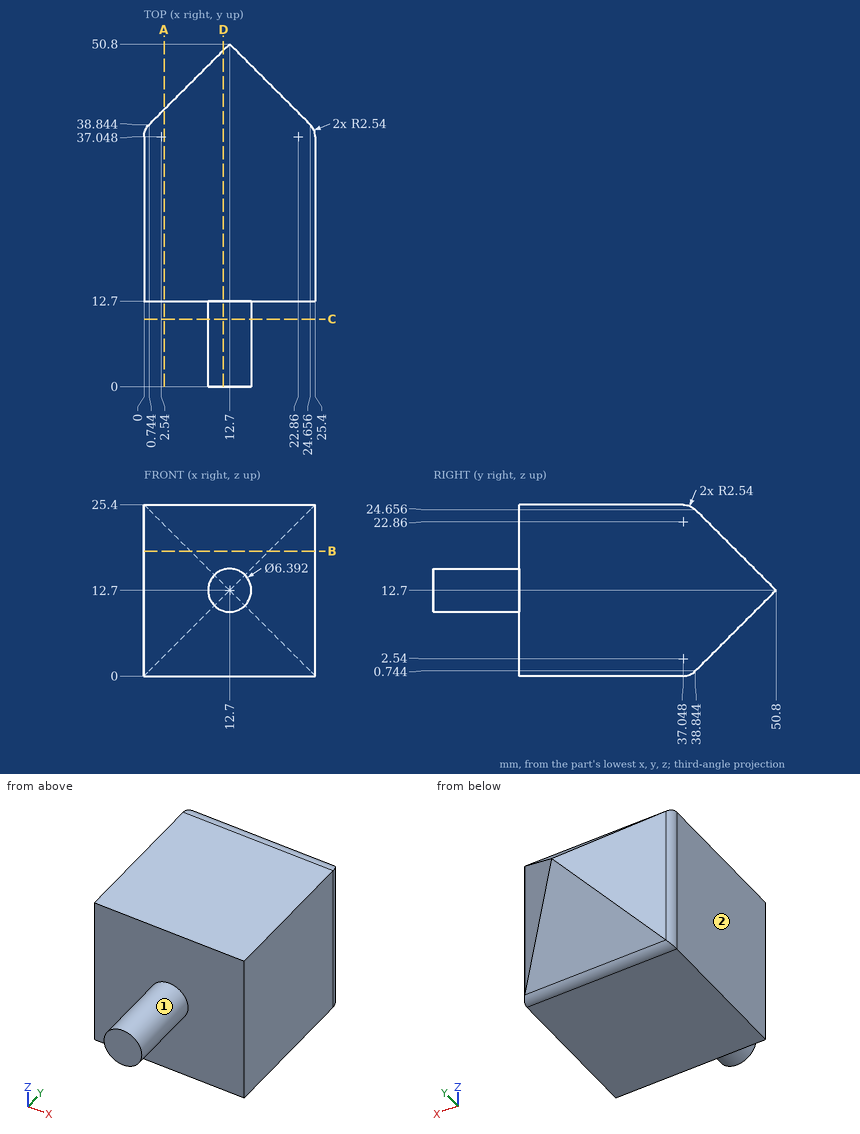
Source: three-view drawing plus pictorial views. Frame: mm from the lowest corner of the part. A direction names the side the tool comes from. Round coordinates to 2 decimals unless told otherwise and drop trailing zeros. Write each loop counter-clockwise with the first axis right and the second up, starting at its lowest first coordinate (ties: lowest second). Pieces come first, ordered by that corner, then holes. Notation, with made-up numbers: M 82.5,-34 L 130.5,-34 A18 ccw 130.5,-23 Z; hole C 9.25,5.25 d1. An arc over 180 degrees is marked long. One line per item, written item: value. Start each with the question number.
Item 1: Section query A-A (x = 3). Return the cut outline in (y, z).
Item 2: Pin query (flat end, axial travel): pin 1 (5 mm diameter, centred on x = 19.5, z = 15, fed in from -Y); pin 2 (1.5 mm diameter, centred on x = 22.5, y = 39, fed in from -Z). Return the tip coordinate at first contact, or that it passes through.
Item 3: Section query D-D (x = 11.75). Return the cut outline in (y, z).
Item 4: Section query B-B (z = 18.5). Return the cut outline in (x, y).
Item 5: Set-up query: the marked faces 1 and 2. Return all of +Z, -Z, +X, -X, +Y, -Y with unobstructed straight access to the full face (end or side cutting, diameter ignored); none if empty.
Item 6: Section query C-C (y = 10). Return the cut outline in (x, z).
Item 7: Ray query, L1, parallel to Y at x = 17, z = 23.5; L2, parallel to Z at x = 10, y = 2; L3, parallel to Y at x = 22.25, z = 1.5. Return the intervals inside material, ascending. Write a range as from..to.
Result set:
1. outline: M 12.7,0 L 37.05,0 A2.54 ccw 38.84,0.74 L 41.1,3 L 41.1,22.4 L 38.84,24.66 A2.54 ccw 37.05,25.4 L 12.7,25.4 Z
2. pin 1: stops at y = 12.7
2. pin 2: stops at z = 0.3
3. outline: M 0,9.65 L 12.7,9.65 L 12.7,0 L 37.05,0 A2.54 ccw 38.84,0.74 L 49.85,11.75 L 49.85,13.65 L 38.84,24.66 A2.54 ccw 37.05,25.4 L 12.7,25.4 L 12.7,15.75 L 0,15.75 Z
4. outline: M 0,12.7 L 25.4,12.7 L 25.4,37.05 A2.54 ccw 24.66,38.84 L 18.5,45 L 6.9,45 L 0.74,38.84 A2.54 ccw 0,37.05 Z
5. face 1: -Y
5. face 2: +Z, -Z, -X, +Y, -Y
6. outline: C 12.7,12.7 d6.39
7. L1: y = 12.7..40
7. L2: z = 10.99..14.41
7. L3: y = 12.7..39.6
